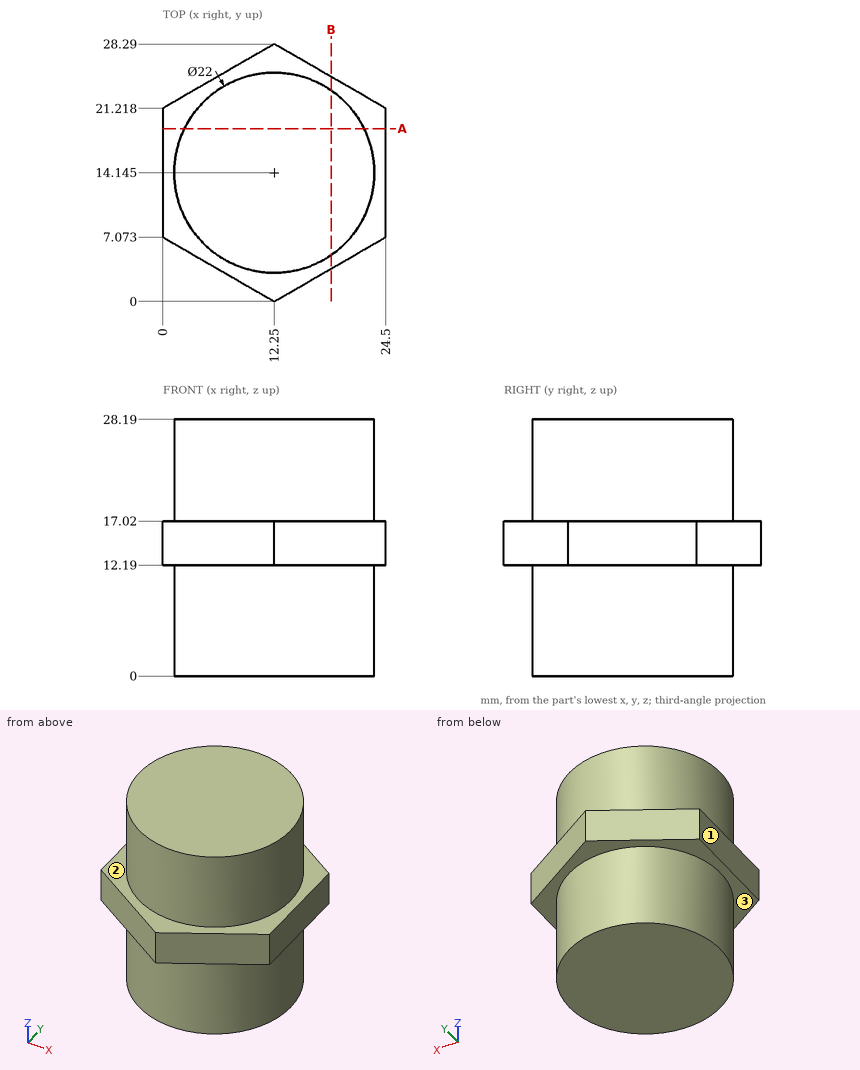
Study the drawing (mm; zero at the part's minimum x, y, z) and answer. A direction names the side the tool comes from. Round coordinates to 2 decimals unless told otherwise and drop trailing zeros. Loops run counter-clockwise (first coordinate to the right, second up) from the corner with the lowest first, then second, coordinate; pieces in that order, holes last. Notation, with made-up numbers: (-12.5, 34) - (15.5, 34) arc R25 ccw to (15.5, 59) - close; hole circle Ø11 at (4.5, 50). An arc over 180 degrees is marked (long way). Use one line per item in the form item = value. Start each with the question number.
1. A tool of negligible diameter and unlimited length cuts with its end or side. For the marked faces 1, 2 and 3, from which of +Z, -Z, +X, -X, +Y, -Y can it reach the whole face along a straight path? Write none if from no direction.
2. Given pin 1 Ø4 at (x, z) = (20, 9.5) entering from +Y; pin 2 Ø1 at (y, z) = (5.5, 19) entering from -X (1 decimal), each flat-ended and moving along its own axis, determine where each tip first touches the part or whether it passes through.
3. Consider line 1 (Z direction, x = 1.5, y = 21.5); line 2 (Y direction, x = 12.25, z = 3) (1 decimal); line 3 (Y direction, x = 9.5, z = 16.25). Determine where each line is inside the solid, lowest interval first. Write a range as [from, to].
4. The part is cut by section A-A on y = 19. Determine the outline of the cut face in (x, z).
5. The part is cut by section B-B on x = 18.5. Determine the outline of the cut face in (y, z), then the cut area to 3 significant figures.
Geometry check:
q1.face_1 = +Z, -Z, -X, +Y, -Y
q1.face_2 = +Z
q1.face_3 = -Z
q2.pin_1 = 23.52
q2.pin_2 = 4.9
q3.line_1 = [12.19, 17.02]
q3.line_2 = [3.1, 25.1]
q3.line_3 = [1.59, 26.7]
q4.outline = (0, 12.19) - (2.38, 12.19) - (2.38, 0) - (22.12, 0) - (22.12, 12.19) - (24.5, 12.19) - (24.5, 17.02) - (22.12, 17.02) - (22.12, 28.19) - (2.38, 28.19) - (2.38, 17.02) - (0, 17.02) - close
q5.outline = (3.61, 12.19) - (5.09, 12.19) - (5.09, 0) - (23.2, 0) - (23.2, 12.19) - (24.68, 12.19) - (24.68, 17.02) - (23.2, 17.02) - (23.2, 28.19) - (5.09, 28.19) - (5.09, 17.02) - (3.61, 17.02) - close
q5.area = 525 mm^2
